Autodesk Inventor part; units mm, degrees
ref_plane "YZ Plane" through (0, 0, 0) normal (1, 0, 0) x (0, 1, 0)
ref_plane "XZ Plane" through (0, 0, 0) normal (0, 1, 0) x (-1, 0, 0)
ref_plane "XY Plane" through (0, 0, 0) normal (0, 0, 1) x (1, 0, 0)
sketch "Sketch1" plane through (0, 0, 0) normal (0, 0, 1) x (1, 0, 0)
  circle A0 centre (0, 0) radius 25.4 construction
  line L0 (-13.75, -13.75) -> (13.75, -13.75) construction
  line L1 (13.75, -13.75) -> (13.75, 13.75) construction
  line L2 (13.75, 13.75) -> (-13.75, 13.75) construction
  line L3 (-13.75, 13.75) -> (-13.75, -13.75) construction
  line L4 (-13.75, -13.75) -> (13.75, 13.75) construction
  line L5 (13.75, -13.75) -> (-13.75, 13.75) construction
  circle A1 centre (0, 0) radius 9.25
  circle A2 centre (-13.75, 13.75) radius 1.7
  circle A3 centre (-13.75, 13.75) radius 2.7
  circle A4 centre (-25.4, 0) radius 1.7
  circle A5 centre (-25.4, 0) radius 3.8
  line L6 (-17, 17) -> (17, 17)
  line L7 (17, 17) -> (17, -17)
  line L8 (17, -17) -> (-17, -17)
  line L9 (-17, -17) -> (-17, 17)
  line L10 (-17, 17) -> (17, -17) construction
  line L11 (17, 17) -> (-17, -17) construction
  line L12 (-25.4, 3.8) -> (-18, 3.8)
  line L13 (-25.4, -3.8) -> (-18, -3.8)
  line L14 (0, 17) -> (0, -17) construction
  line L15 (-17, 0) -> (17, 0) construction
  circle A6 centre (25.4, 0) radius 1.7
  circle A7 centre (25.4, 0) radius 3.8
  line L16 (25.4, 3.8) -> (18, 3.8)
  line L17 (25.4, -3.8) -> (18, -3.8)
  circle A8 centre (13.75, 13.75) radius 1.7
  circle A9 centre (13.75, 13.75) radius 2.7
  circle A10 centre (-13.75, -13.75) radius 1.7
  circle A11 centre (-13.75, -13.75) radius 2.7
  circle A12 centre (13.75, -13.75) radius 2.7
  circle A13 centre (13.75, -13.75) radius 1.7
  line L18 (-18, 18) -> (18, 18)
  line L19 (18, 18) -> (18, -18)
  line L20 (18, -18) -> (-18, -18)
  line L21 (-18, -18) -> (-18, 18)
  line L22 (-18, 18) -> (18, -18) construction
  line L23 (18, 18) -> (-18, -18) construction
  point P0 (-17, 3.8)
  point P1 (-17, -3.8)
  point P2 (17, 3.8)
  point P3 (17, -3.8)
  dimension "d0" = 50.8
  dimension "d1" = 27.5
  dimension "d2" = 27.5
  dimension "d3" = 18.5
  dimension "d4" = 3.4
  dimension "d5" = 5.4
  dimension "d6" = 3.4
  dimension "d7" = 7.6
  dimension "d8" = 34
  dimension "d9" = 34
  dimension "d10" = 36
  dimension "d11" = 36
extrude "Extrusion1" add sketch "Sketch1" against normal blind 10 contours A3 | L21 L18 L19 L20 | A9 | A11 | A12
extrude "Extrusion2" add sketch "Sketch1" against normal blind 2.2 contours L6 L7 L8 L9
fillet "Fillet1" radius 0.6 8 edges at (18, 0, 0) (0, 18, 0) (-18, 0, 0) (0, -18, 0) (18, 18, -5) (-18, 18, -5) (-18, -18, -5) (18, -18, -5)
equation "\"d9\" = d8"
properties part number "cameraTop"
Geometry check sheet. Reference: the model listing, model coordinates, mm. A direction names the side the tool comes from. Round coordinates to 2 decimals unless told otherwise and drop trailing zeros. Loops run counter-clockwise (first coordinate to the right, second up) from the corner with the lowest first, then second, coordinate; pieces in that order, holes last.
Item 1: Gauge pin test, flat end, axial feed: pin 1 (10 mm diameter, centred on x = -4.5, y = -10, fed in from -Z). Record the tip position at first contact, or that the pin passes through.
Item 2: Mould release check, pull along X, two halves, no side actions. Record for faces 3 (the flat face through (18, 0, -5)), 4 (the flat face through (0, 18, -5)), 5 (the flat face through (-17, 0, -6)): pulls with the +X half, pulls with the -X half, needs draft (parallel to the pull), parting line crosses it, or undercut.
Item 3: Cross-section at C-C on y = -13.75. Record the boundary of the cut face in (x, z), then the cut area to 3 significant figures.
Item 4: Access from +Z, -Z, +X, -X, +Y, -Y to the whole of each face (thin tool, end or side, straight path). Record for faces 1 (the cylindrical face through (15.202, 16.027, -6.045)), 2 (the flat face through (-12, 13, -10)).
Item 5: Thickness scan on line 1 (Y direction, x = 13.75, z = -4); line 2 (X direction, y = -4, z = -4.5). Record the ranges inside material, lowest first.
Item 6: Cross-section at B-B on x = -3. Record the boundary of the cut face in (y, z).
Item 7: Cross-section at A-A on z = -4.5. Count the separate pieces of the cut face and the enclosed holes in it, then the cut area to 3 significant figures.
Answer sheet:
1. pin 1: stops at z = -2.2
2. face 3: pulls with the +X half
2. face 4: needs draft
2. face 5: undercut
3. outline: (-18, -10) - (-17, -10) - (-17, -2.2) - (-16.45, -2.2) - (-16.45, -10) - (-15.45, -10) - (-15.45, 0) - (-17.4, 0) arc R0.6 ccw to (-18, -0.6) - close; (-12.05, -10) - (-11.05, -10) - (-11.05, -2.2) - (11.05, -2.2) - (11.05, -10) - (12.05, -10) - (12.05, 0) - (-12.05, 0) - close; (15.45, -10) - (16.45, -10) - (16.45, -2.2) - (17, -2.2) - (17, -10) - (18, -10) - (18, -0.6) arc R0.6 ccw to (17.4, 0) - (15.45, 0) - close
3. area: 111 mm2
4. face 1: -Z
4. face 2: -Z, +X, -X, +Y, -Y
5. line 1: y = -18 to -17, -16.45 to -15.45, -12.05 to -11.05, 11.05 to 12.05, 15.45 to 16.45, 17 to 18
5. line 2: x = -18 to -17, 17 to 18
6. outline: (-18, -10) - (-17, -10) - (-17, -2.2) - (-8.75, -2.2) - (-8.75, 0) - (-17.4, 0) arc R0.6 ccw to (-18, -0.6) - close; (8.75, -2.2) - (17, -2.2) - (17, -10) - (18, -10) - (18, -0.6) arc R0.6 ccw to (17.4, 0) - (8.75, 0) - close
7. separate pieces: 5
7. enclosed holes: 5
7. area: 195 mm2
